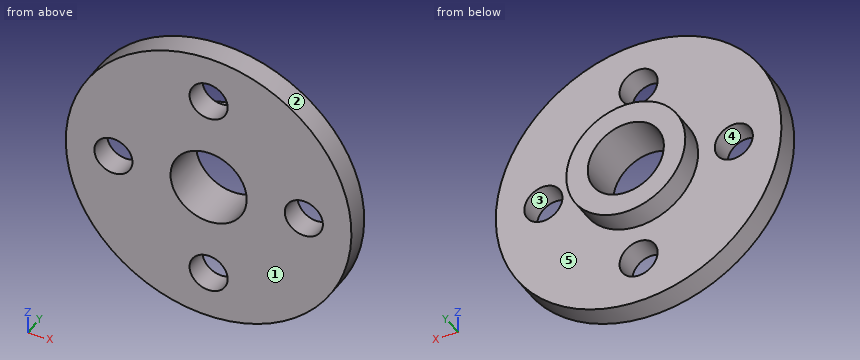
from build123d import *

# Parameters (mm, degrees)
SKETCH1_R           = 30
SKETCH1_R_2         = 4
SKETCH1_R_3         = 12.5
BOSS_EXTRUDE1_DEPTH = 5
SKETCH1_6_R         = 12.5
SKETCH1_6_R_2       = 8
BOSS_EXTRUDE2_DEPTH = 10


with BuildPart() as part:
    # Sketch1 → Boss-Extrude1 (new body)
    with BuildSketch(Plane(origin=(0, 0, 0), x_dir=(1, 0, 0), z_dir=(0, 1, 0))):
        with Locations(Location((0, 0, 0), (0, 0, 270))):
            Circle(SKETCH1_R)
        with Locations(Location((0, 20, 0), (0, 0, 270))):
            Circle(SKETCH1_R_2, mode=Mode.SUBTRACT)
        with Locations(Location((20, 0, 0), (0, 0, 270))):
            Circle(SKETCH1_R_2, mode=Mode.SUBTRACT)
        with Locations(Location((0, -20, 0), (0, 0, 270))):
            Circle(SKETCH1_R_2, mode=Mode.SUBTRACT)
        with Locations(Location((-20, 0, 0), (0, 0, 270))):
            Circle(SKETCH1_R_2, mode=Mode.SUBTRACT)
        with Locations(Location((0, 0, 0), (0, 0, 270))):
            Circle(SKETCH1_R_3, mode=Mode.SUBTRACT)
    extrude(amount=BOSS_EXTRUDE1_DEPTH)

    # Sketch1_6 → Boss-Extrude2 (add)
    with BuildSketch(Plane(origin=(0, 0, 0), x_dir=(1, 0, 0), z_dir=(0, 1, 0))):
        with Locations(Location((0, 0, 0), (0, 0, 270))):
            Circle(SKETCH1_6_R)
        with Locations(Location((0, 0, 0), (0, 0, 270))):
            Circle(SKETCH1_6_R_2, mode=Mode.SUBTRACT)
    extrude(amount=BOSS_EXTRUDE2_DEPTH)


solid = part.part
Work out the finished part from the listing and answer in its coordinate system (mm). Face numbers are marked on the shaded views. A direction names the side the tool comes from. Round coordinates to 2 decimals unless told otherwise and drop trailing zeros. Write each loop counter-clockwise with the first axis right and the second up, starting at its lowest first coordinate (ties: lowest second). Pieces come first, ordered by that corner, then holes. Notation, with made-up numbers: (42, 31) - (85, 31) arc R25 ccw to (85, 68) - close; hole circle Ø3 at (46, 44). An arc over 180 degrees is marked (long way). Answer in a Markdown table with one row per item. Add a question column.
1. For the marked faces 4 and 5, determine the directions among +Z, -Z, +X, -X, +Y, -Y from which every point of the face is accessible in a straight line to the end or side of a thin tool.
2. A cutting plane is placed at A-A, the plane z = 0. Determine the outline of the cut face in (x, y).
3. A cutting plane is placed at B-B, the plane x = 0. Determine the outline of the cut face in (y, z).
4. A cutting plane is placed at D-D, the plane x = 20. Determine the outline of the cut face in (y, z), and give its area (3 significant figures).
5. Given pin 1 (6.5 mm diameter, centred on x = 0, z = 20, fed in from -Y); pin 2 (2 mm diameter, centred on x = -23, z = -2.5, fed in from +Y); pin 3 (2 mm diameter, centred on x = 16, y = 4.5, fed in from +Z); pin 4 (2 mm diameter, centred on x = 20.5, y = 2.5, fed in from -Z), each flat-ended and moving along its own axis, determine where each tip first touches the part or whether it passes through.
6. The mould has two halves that part along Z. Classify the marked faces 1, 2 and 3: +Z half, -Z half, draft (parallel to the pull), parting line (faces both ways), or undercut.
7. A cutting plane is placed at C-C, the plane y = 3. Determine the outline of the cut face in (x, z), and give its area (3 significant figures).
8. Find the intervals of material crossed by line 1 along X through (y, z) = (3.45, 0); line 2 along X through (y, z) = (3.75, -2); line 3 along X through (y, z) = (6.25, 0), in increasing order. Write a range as from..to.
Worked out:
| question | item | result |
|---|---|---|
| 1 | face 4 | +Y, -Y |
| 1 | face 5 | +Y |
| 2 | outline | (-30, 0) - (-24, 0) - (-24, 5) - (-30, 5) - close; (-16, 0) - (-8, 0) - (-8, 10) - (-12.5, 10) - (-12.5, 5) - (-16, 5) - close; (8, 0) - (16, 0) - (16, 5) - (12.5, 5) - (12.5, 10) - (8, 10) - close; (24, 0) - (30, 0) - (30, 5) - (24, 5) - close |
| 3 | outline | (0, -30) - (5, -30) - (5, -24) - (0, -24) - close; (0, -16) - (5, -16) - (5, -12.5) - (10, -12.5) - (10, -8) - (0, -8) - close; (0, 8) - (10, 8) - (10, 12.5) - (5, 12.5) - (5, 16) - (0, 16) - close; (0, 24) - (5, 24) - (5, 30) - (0, 30) - close |
| 4 | outline | (0, -22.36) - (5, -22.36) - (5, -4) - (0, -4) - close; (0, 4) - (5, 4) - (5, 22.36) - (0, 22.36) - close |
| 4 | area | 184 mm^2 |
| 5 | pin 1 | through |
| 5 | pin 2 | y = 5 |
| 5 | pin 3 | z = 25.98 |
| 5 | pin 4 | z = -22.8 |
| 6 | face 1 | draft |
| 6 | face 2 | parting line |
| 6 | face 3 | undercut |
| 7 | outline | circle Ø60 at (0, 0); hole circle Ø8 at (-20, 0); hole circle Ø16 at (0, 0); hole circle Ø8 at (0, -20); hole circle Ø8 at (0, 20); hole circle Ø8 at (20, 0) |
| 7 | area | 2,430 mm^2 |
| 8 | line 1 | -30..-24, -16..-8, 8..16, 24..30 |
| 8 | line 2 | -29.93..-23.46, -16.54..-7.75, 7.75..16.54, 23.46..29.93 |
| 8 | line 3 | -12.5..-8, 8..12.5 |
